Read the model definition and answer for the solid it produces. Units are mm, in the model's axes. A direction names the side the tool comes from. Give positions to 0.01 mm unless a question says otherwise; leave off trailing zeros. Order: outer loops, then holes, each group sorted by start corner. A loop starts at its lowest first (then second) coordinate and runs counter-clockwise, first axis right, second up. Notation, with made-up numbers: (85.25, -28.5) -> (98.25, -28.5) arc R13 ccw to (98.25, -16.5) -> close; hole circle Ø3 at (27, 87). An arc over 180 degrees is marked (long way). Answer as CSV lines item,"result". Start each with the question number.
1) Straight lines are drawn through the part: L1, parallel to X at y = 0.1, z = -16; L2, parallel to Z at x = -1, y = 1.1; L3, parallel to X at y = 0.1, z = 17. For each, find the intervals that lie inside material, in ascending order. Write a range as from..to.
2) Find section A-A (x = 12). Determine the outline of the cut face in (y, z).
3) Find section B-B (z = -6). Determine the outline of the cut face in (x, y).
4) Flat-ended cylindrical pins translate along their axes: pin 1 Ø1 at (x, y) = (17.5, 1) entering from +Z; pin 2 Ø1 at (y, z) = (1, 0) entering from -X (3 decimals); pin 3 Ø1 at (x, y) = (-18.5, 0.5) entering from -Z. Find the tip coordinate at first contact, or state that the pin passes through.
5) For faces 1 (the face through (8.123, 1.014, 16.069)), 2 (the face through (-17.707, 0.986, 10.38)), determine the directions among +Z, -Z, +X, -X, +Y, -Y from which every point of the face is accessible in a straight line to the end or side of a thin tool.
6) The mould has two halves that part along X. Classify faces 3 (the face through (-0.136, 0.986, -20.525)), 4 (the face through (-15.525, 1, 0)), 5 (the face through (9.855, 1.014, -15.069)): +X half, -X half, draft (parallel to the pull), parting line (faces both ways), or undercut.
Autodesk Inventor part; units mm, degrees
ref_plane "YZ Plane" through (0, 0, 0) normal (1, 0, 0) x (0, 1, 0)
ref_plane "XZ Plane" through (0, 0, 0) normal (0, 1, 0) x (-1, 0, 0)
ref_plane "XY Plane" through (0, 0, 0) normal (0, 0, 1) x (1, 0, 0)
sketch "Sketch1" plane through (0, 0, 0) normal (0, 1, 0) x (-1, 0, 0)
  circle A0 centre (0, 0) radius 20.525
  circle A1 centre (0, 0) radius 10.525
  dimension "d0" = 41.05
  dimension "d1" = 21.05
extrude "Extrusion1" add sketch "Sketch1" along normal blind 2
sketch "Sketch2" plane through (0, 2, 0) normal (0, 1, 0) x (1, 0, 0)
  line L0 (-25.525, -1) -> (-15.525, -1)
  line L1 (-15.525, -1) -> (-15.525, 1)
  line L2 (-15.525, 1) -> (-25.525, 1)
  line L3 (-25.525, 1) -> (-25.525, -1)
  point P0 (0, 0)
  dimension "d4" = 1
  dimension "d5" = 2
  dimension "d6" = 10
  dimension "d7" = 15.525
extrude "Extrusion2" cut sketch "Sketch2" against normal blind 2
pattern_circular "Circular Pattern1" count 6 over 360 about axis through (0, -10, 0) along (0, 1, 0) of "Extrusion2"
sketch "Sketch3" plane through (0, 2, 0) normal (0, 1, 0) x (1, 0, 0)
  circle A0 centre (-2.5981, -1.5) radius 10
  line L0 (-2.5981, -1.5) -> (0, 0) construction
  line L1 (-34.9729, 0) -> (29.7462, 0)
  dimension "d13" = 20
  dimension "d14" = 30
  dimension "d15" = 1.5
extrude "Extrusion3" cut sketch "Sketch3" against normal blind 2
pattern_circular "Circular Pattern2" count 6 over 360 about axis through (0, -10, 0) along (0, 1, 0) of "Extrusion3"
fillet "Fillet1" radius 5 6 edges at (-6.2425, 1, -10.8123) (-12.4849, 1, 0) (6.2425, 1, -10.8123) (-6.2425, 1, 10.8123) (6.2425, 1, 10.8123) (12.4849, 1, 0)
properties part number "Ring_n5"
Findings below:
1,L1,"-12.86..-10.39, -8.08..8.08, 10.39..12.86"
1,L2,"-20.5..-12.95, 12.95..20.5"
1,L3,"-11.5..-10.97, -8.66..8.66, 10.97..11.5"
2,outline,"(0, -16.65) -> (2, -16.65) -> (2, -4.91) -> (0, -4.91) -> close; (0, 4.91) -> (2, 4.91) -> (2, 16.65) -> (0, 16.65) -> close"
3,outline,"(-19.63, 0) -> (-11.53, 0) -> (-11.53, 2) -> (-19.63, 2) -> close; (11.53, 0) -> (19.63, 0) -> (19.63, 2) -> (11.53, 2) -> close"
4,pin 1,"z = 11.5"
4,pin 2,"x = -15.525"
4,pin 3,"z = -9.86"
5,face 1,"+Y, -Y"
5,face 2,"+Z, -X, +Y, -Y"
6,face 3,"parting line"
6,face 4,"-X half"
6,face 5,"undercut"
